Can you work these out from the drawing? Everything is in mm from the part's minimum corner. A direction names the side the tool comes from. Give positions to 0.01 mm unless a question says otherwise; leave off trailing zeros. Loops run counter-clockwise (first coordinate to the right, second up) from the corner with the lowest first, then second, coordinate; pieces in that order, holes last.
Q1. If we section it at A-A (y = 0.45): Please give me the cut outline in (x, z).
Q2. For the marked faces 4 and 5, which set-ups out of +Z, -Z, +X, -X, +Y, -Y let a thin tool reach every point of the face, with its end or its side?
Q3. Will these pins go through, and if not, where does the flat tip stop? P1, Ø1.5, axis at x = 5.5, y = 2, coming from the +Z side; P2, Ø4, axis at x = 9.5, z = 2, coming from the +Y side; P3, Ø3, axis at y = 5, z = 4.5, coming from the -X side (1 decimal).
Q4. We'd pull the mould along X, two halves only. Please class the marked faces 1, 2 and 3: +X half, -X half, draft (parallel to the pull), parting line (faces both ways), or undercut.
Q5. If we section it at D-D (y = 2.5): Please give me the cut outline in (x, z).
Q6. I need wall thicknesses on line 1 (X direction, y = 1.75, z = 3.25) (1 decimal); line 2 (X direction, y = 0.65, z = 7); line 3 (Z direction, x = 6.25, y = 2.8). Which ranges of each line are inside material? Lowest first, please.
Q7. If we section it at B-B (x = 5): Please give me the cut outline in (y, z) (1 decimal), plus the area to 3 significant figures.
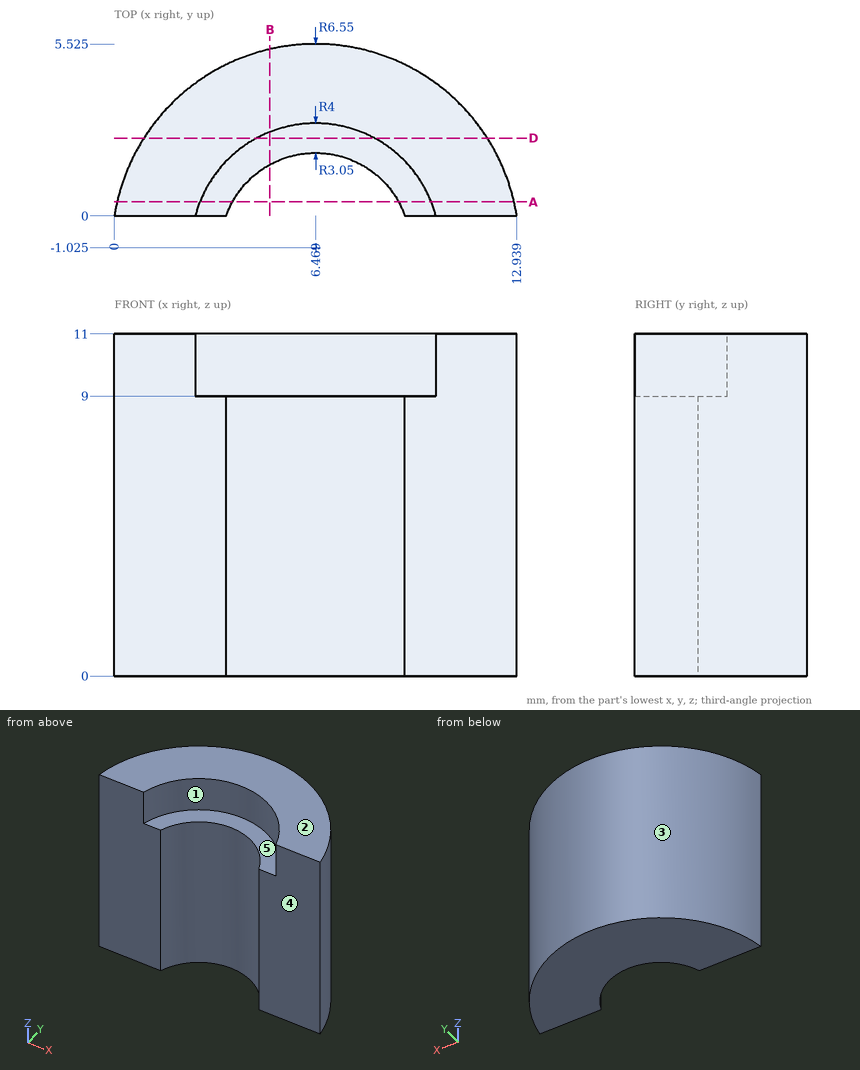
Check sheet entries:
1. outline: (0.09, 0) - (3.8, 0) - (3.8, 9) - (2.75, 9) - (2.75, 11) - (0.09, 11) - close; (9.14, 0) - (12.85, 0) - (12.85, 11) - (10.19, 11) - (10.19, 9) - (9.14, 9) - close
2. face 4: +Z, -Z, +X, -X, -Y
2. face 5: +Z, -Y
3. P1: stops at z = 9
3. P2: stops at y = 5.44
3. P3: stops at x = 1.7
4. face 1: undercut
4. face 2: draft
4. face 3: parting line
5. outline: (0.95, 0) - (11.99, 0) - (11.99, 11) - (8.36, 11) - (8.36, 9) - (4.58, 9) - (4.58, 11) - (0.95, 11) - close
6. line 1: x = 0.5 to 5.2, 7.7 to 12.4
6. line 2: x = 0.14 to 3.92, 9.02 to 12.8
6. line 3: z = 0 to 9
7. outline: (1.6, 0) - (5.4, 0) - (5.4, 11) - (2.7, 11) - (2.7, 9) - (1.6, 9) - close
7. area: 38.7 mm2
